Read the model definition and answer for the solid it produces. Units are mm, in the model's axes. A direction names the side the tool comes from. Round coordinates to 2 decimals unless told otherwise and drop trailing zeros. Write each loop counter-clockwise with the first axis right and the second up, starting at its lowest first coordinate (ties: lowest second). Pieces come first, ordered by that corner, then holes. Notation, with made-up numbers: (9.5, -32) - (67.5, -32) arc R37 ccw to (67.5, 4) - close; hole circle Ø3 at (10, 31). An arc over 180 degrees is marked (long way). Use one line per item in the form item = value. Start each with the question number.
1) The part is cut by section A-A, the plane x = 0. Give the vertices of the cut face in (y, z) (3 decimals), plus the area to 3 significant figures.
2) Consider line 1 along Y through (x, z) = (-29.5, -27.5) (3 decimals); line 2 along Y through (x, z) = (33.5, -28.5) (3 decimals); line 3 along X through (y, z) = (2.5, -35). Determine where each line is inside the solid, lowest interval first. Write a range as from..to.
3) For faces 1 (the face through (-41, 0, -31)), 2 (the face through (28.978, -1.565, -10.165)), 3 (the face through (-59.417, 1.565, -22.568)), determine the directions among +Z, -Z, +X, -X, +Y, -Y from which every point of the face is accessible in a straight line to the end or side of a thin tool.
4) The part is cut by section B-B, the plane y = -1. Count the separate pieces of the cut face and the enclosed holes in it, plus the area to 3 significant figures.
5) For a pull along Z with two mould halves and no side action, classify faces 4 (the face through (-10.188, 1.565, -34.335)), 5 (the face through (-25.475, 1.565, -8.973)), 6 (the face through (-38, 0, 28)), 7 (the face through (-41.86, -1.57, 45.87)) as released by +Z, released by -Z, zero draft, split by the parting line, or undercut.
6) Each of these flat-tipped pins is pushed along its axis until it touches: pin 1 (10 mm diameter, centred on x = -39.56, z = -49.67, fed in from -Y); pin 2 (4 mm diameter, centred on x = -74.33, z = -21.98, fed in from -Y); pin 3 (3 mm diameter, centred on y = -1, z = -44, fed in from -X); pin 4 (10 mm diameter, centred on x = 28.07, z = -23.59, fed in from +Y). Where does it stop, or does it pass through?
from build123d import *

# Parameters (mm, degrees)
F0_R     = 3.175
F0_R_2   = 3.9751
F1_DEPTH = 3.175
F2_R     = 3.175
F2_R_2   = 3.9751
F3_DEPTH = 3.175


with BuildPart() as f1:
    # F0 (on Front) → F1 (new body)
    with BuildSketch(Plane.XZ):
        with BuildLine():
            ThreePointArc((-12.043522, -10.342591), (-11.221295, 11.229344), (10.351223, 12.036104))
            Line((10.351223, 12.036104), (-37.153666, 52.890995))
            ThreePointArc((-37.153666, 52.890995), (-34.655856, 49.244679), (-33.776906, 44.913152))
            ThreePointArc((-33.776906, 44.913152), (-48.773737, 34.501638), (-53.286401, 52.19176))
            Line((-53.286401, 52.19176), (-82.326466, 18.689574))
            ThreePointArc((-82.326466, 18.689574), (-73.55409, 20.927364), (-68.391112, 13.490568))
            ThreePointArc((-68.391112, 13.490568), (-69.108992, 10.191933), (-71.132779, 7.489966))
            Line((-71.132779, 7.489966), (-52.061254, 24.003719))
            ThreePointArc((-52.061254, 24.003719), (-46.270956, 25.922078), (-40.825712, 23.173085))
            Line((-40.825712, 23.173085), (-12.043522, -10.342591))
        make_face()
        with BuildLine():
            ThreePointArc((-33.776906, 44.913152), (-34.655856, 49.244679), (-37.153666, 52.890995))
            ThreePointArc((-37.153666, 52.890995), (-45.370599, 56.015229), (-53.286401, 52.19176))
            ThreePointArc((-53.286401, 52.19176), (-48.773737, 34.501638), (-33.776906, 44.913152))
        make_face()
        with Locations((-44.889406, 44.913152)):
            Circle(F0_R, mode=Mode.SUBTRACT)
        with BuildLine():
            ThreePointArc((-68.391112, 13.490568), (-73.55409, 20.927364), (-82.326466, 18.689574))
            ThreePointArc((-82.326466, 18.689574), (-81.942756, 7.879392), (-71.132779, 7.489966))
            ThreePointArc((-71.132779, 7.489966), (-69.108992, 10.191933), (-68.391112, 13.490568))
        make_face()
        with Locations((-76.328612, 13.490568)):
            Circle(F0_R, mode=Mode.SUBTRACT)
        with BuildLine():
            ThreePointArc((-8.037107, -13.690162), (7.887539, -13.776877), (15.875, 0))
            ThreePointArc((15.875, 0), (15.152816, 4.733687), (13.051972, 9.036684))
            ThreePointArc((13.051972, 9.036684), (11.79731, 10.622576), (10.351223, 12.036104))
            ThreePointArc((10.351223, 12.036104), (-11.221295, 11.229344), (-12.043522, -10.342591))
            Line((-12.043522, -10.342591), (-8.037107, -13.690162))
        make_face()
        Circle(F0_R_2, mode=Mode.SUBTRACT)
        with BuildLine():
            ThreePointArc((13.051972, 9.036684), (15.152816, 4.733687), (15.875, 0))
            ThreePointArc((15.875, 0), (7.887539, -13.776877), (-8.037107, -13.690162))
            Line((-8.037107, -13.690162), (28.786313, -44.458066))
            ThreePointArc((28.786313, -44.458066), (28.068027, -28.058597), (44.464791, -28.836207))
            Line((44.464791, -28.836207), (13.051972, 9.036684))
        make_face()
        with BuildLine():
            ThreePointArc((25.820386, -25.834045), (26.851412, -20.656097), (31.241044, -23.589575))
            ThreePointArc((31.241044, -23.589575), (29.280676, -26.523053), (25.820386, -25.834045))
        make_face(mode=Mode.SUBTRACT)
        with BuildLine():
            ThreePointArc((47.024025, -35.930522), (46.364654, -32.159614), (44.464791, -28.836207))
            ThreePointArc((44.464791, -28.836207), (28.068027, -28.058597), (28.786313, -44.458066))
            ThreePointArc((28.786313, -44.458066), (40.618368, -45.996965), (47.024025, -35.930522))
        make_face()
        with Locations((35.911525, -35.930522)):
            Circle(F0_R, mode=Mode.SUBTRACT)
    extrude(amount=F1_DEPTH)

    # F2 (on Front) → F3 (join)
    with BuildSketch(Plane.XZ):
        with BuildLine():
            ThreePointArc((11.640623, -10.79405), (-9.929683, -12.386162), (-13.067664, 9.013978))
            Line((-13.067664, 9.013978), (-38.234496, -27.47066))
            ThreePointArc((-38.234496, -27.47066), (-43.332686, -30.774036), (-49.275206, -29.512973))
            Line((-49.275206, -29.512973), (-69.846496, -15.426666))
            ThreePointArc((-69.846496, -15.426666), (-67.309692, -18.274033), (-66.393606, -21.975878))
            ThreePointArc((-66.393606, -21.975878), (-71.142789, -29.24489), (-79.707254, -27.815479))
            Line((-79.707254, -27.815479), (-47.089017, -57.845007))
            ThreePointArc((-47.089017, -57.845007), (-48.001609, -42.439933), (-32.638988, -40.977391))
            ThreePointArc((-32.638988, -40.977391), (-29.551811, -44.845089), (-28.44991, -49.669565))
            ThreePointArc((-28.44991, -49.669565), (-29.217432, -53.727777), (-31.413974, -57.2254))
            Line((-31.413974, -57.2254), (11.640623, -10.79405))
        make_face()
        with BuildLine():
            ThreePointArc((-23.521714, -33.517023), (-25.318293, -36.377194), (-28.674835, -36.000501))
            ThreePointArc((-28.674835, -36.000501), (-28.075136, -30.656851), (-23.521714, -33.517023))
        make_face(mode=Mode.SUBTRACT)
        with BuildLine():
            ThreePointArc((-66.393606, -21.975878), (-67.309692, -18.274033), (-69.846496, -15.426666))
            ThreePointArc((-69.846496, -15.426666), (-80.541531, -17.032749), (-79.707254, -27.815479))
            ThreePointArc((-79.707254, -27.815479), (-71.142789, -29.24489), (-66.393606, -21.975878))
        make_face()
        with Locations((-74.331106, -21.975878)):
            Circle(F2_R, mode=Mode.SUBTRACT)
        with BuildLine():
            ThreePointArc((11.640623, -10.79405), (14.77854, -5.797445), (15.875, 0))
            ThreePointArc((15.875, 0), (4.720512, 15.156926), (-13.067664, 9.013978))
            ThreePointArc((-13.067664, 9.013978), (-9.929683, -12.386162), (11.640623, -10.79405))
        make_face()
        Circle(F2_R_2, mode=Mode.SUBTRACT)
        with BuildLine():
            ThreePointArc((-47.089017, -57.845007), (-39.123496, -60.773394), (-31.413974, -57.2254))
            ThreePointArc((-31.413974, -57.2254), (-29.217432, -53.727777), (-28.44991, -49.669565))
            ThreePointArc((-28.44991, -49.669565), (-29.551811, -44.845089), (-32.638988, -40.977391))
            ThreePointArc((-32.638988, -40.977391), (-48.001609, -42.439933), (-47.089017, -57.845007))
        make_face()
        with BuildLine():
            ThreePointArc((-36.38741, -49.669565), (-42.422581, -51.047987), (-37.58429, -47.186087))
            ThreePointArc((-37.58429, -47.186087), (-36.702239, -48.291143), (-36.38741, -49.669565))
        make_face(mode=Mode.SUBTRACT)
    extrude(amount=-F3_DEPTH)


solid = f1.part
Geometry results:
q1.outline = (-3.175, -20.406) - (0, -20.406) - (0, -23.348) - (3.175, -23.348) - (3.175, -3.975) - (-3.175, -3.975) - close; (-3.175, 3.975) - (3.175, 3.975) - (3.175, 15.875) - (0, 15.875) - (0, 20.938) - (-3.175, 20.938) - close
q1.area = 205 mm2
q2.line_1 = 0..3.175
q2.line_2 = -3.175..0
q2.line_3 = -71.9..-29.5, -23.89..-10.8
q3.face_1 = -Z, -X, -Y
q3.face_2 = +Z, +X, +Y, -Y
q3.face_3 = +Z, +Y, -Y
q4.separate_pieces = 1
q4.enclosed_holes = 5
q4.area = 4,040 mm2
q5.face_4 = released by -Z
q5.face_5 = released by +Z
q5.face_6 = zero draft
q5.face_7 = undercut
q6.pin_1 = 0
q6.pin_2 = through
q6.pin_3 = -63.34
q6.pin_4 = 0
